Design review of the part built by this model. Coordinates are the model's own, in mm. Face numbers are marked on the shaded views. A direction names the side the tool comes from. Round coordinates to 2 decimals unless told otherwise and drop trailing zeros. Loops run counter-clockwise (first coordinate to the right, second up) from the corner with the lowest first, then second, coordinate; pieces in that order, holes last. Notation, with made-up numbers: M 27,6 L 59,6 A30 ccw 59,33 Z; hole C 84,71.5 d2. An arc over 180 degrees is marked long. Use a Markdown table: item, result.
Autodesk Inventor part; units mm, degrees
ref_plane "YZ Plane" through (0, 0, 0) normal (1, 0, 0) x (0, 1, 0)
ref_plane "XY Plane" through (0, 0, 0) normal (0, 0, 1) x (1, 0, 0)
sketch "Sketch2" plane through (0, 0, 0) normal (0, 0, 1) x (1, 0, 0)
  circle A0 centre (0, 0) radius 76.2
  dimension "d7" = 152.4
extrude "Extrusion2" add sketch "Sketch2" along normal blind 88.9
chamfer "Chamfer1" distance 19.05 angle 30 1 edges at (-76.2, 0, 88.9) measured on face at (-0.8389, -20.4706, 88.9)
chamfer "Chamfer2" distance 19.05 angle 30 1 edges at (-76.2, 0, 0) measured on face at (-0.8389, -20.4706, 0)
ref_plane "Work Plane1" through (0, -76.2, 0) normal (0, 1, 0) x (-1, 0, 0)
sketch "Sketch10" plane through (0, -76.2, 0) normal (0, 1, 0) x (-1, 0, 0)
  line L0 (88.9, 77.9015) -> (-88.9, 77.9015)
  line L1 (-88.9, 77.9015) -> (-88.9, 10.9985)
  line L2 (-88.9, 10.9985) -> (88.9, 10.9985)
  line L3 (88.9, 10.9985) -> (88.9, 77.9015)
  line L4 (-76.2, 10.9985) -> (76.2, 10.9985) construction
  line L5 (76.2, 77.9015) -> (-76.2, 77.9015) construction
  line L6 (0, -18.1203) -> (0, 108.7218) construction
  dimension "d46" = 88.9
  dimension "d47" = 88.9
extrude "Extrusion11" add sketch "Sketch10" along normal mid plane 76.2
properties part number "transmission_box_l_to_r"
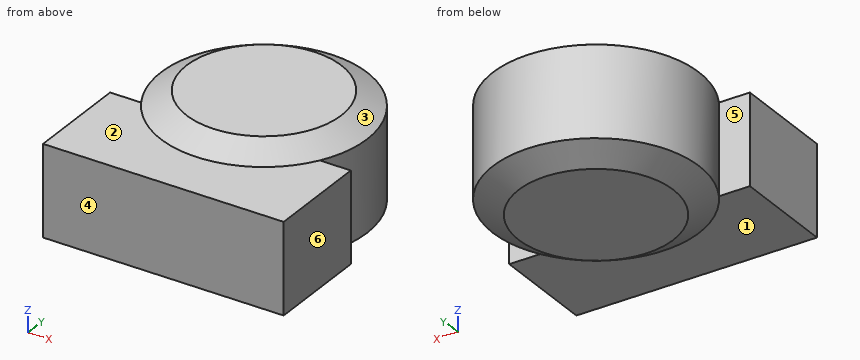
1. The part is to be moulded in two halves that separate along Y. For the marked faces 4, 5 and 6, say which applies: pulls with the +Y half, pulls with the -Y half, needs draft (parallel to the pull), parting line crosses it, or undercut.
Check values:
| item | result |
|---|---|
| face 4 | pulls with the -Y half |
| face 5 | undercut |
| face 6 | needs draft |
2. Take a section at C-C on z = 18.5. Give the boundary of the cut face in (x, y).
Check values:
| item | result |
|---|---|
| outline | M -88.9,-114.3 L 88.9,-114.3 L 88.9,-38.1 L 65.99,-38.1 A76.2 ccw long -65.99,-38.1 L -88.9,-38.1 Z |
3. Insertion check: pin 1 (5 mm diameter, centred on x = -14, z = 71.5, fed in from +Y); pin 2 (3 mm diameter, centred on y = -26, z = 24, fed in from +X); pin 3 (1.5 mm diameter, centred on x = 55, y = -71.5, fed in from -Z). Each pin has a flat end and moves straight along its axis. Give the tip position at first contact, or say it passes through.
Check values:
| item | result |
|---|---|
| pin 1 | stops at y = 75.33 |
| pin 2 | stops at x = 72.15 |
| pin 3 | stops at z = 11 |
4. Wall thickness on line 1 along Y through (x, z) = (-1.5, 24.5); line 2 along Y through (x, z) = (-80, 23); line 3 along X through (y, z) = (1.5, 22.5): over which ranges is each line inside the solid? List them lowest first. Write a range as from..to.
Check values:
| item | result |
|---|---|
| line 1 | y = -114.3..76.19 |
| line 2 | y = -114.3..-38.1 |
| line 3 | x = -76.19..76.19 |
5. Machinability: for the marked faces 1, 2 and 3, which of the approach directions +Z, -Z, +X, -X, +Y, -Y give a long, thin tool a straight path to every point of the face, cutting with its end or side? Answer none if there is none.
Check values:
| item | result |
|---|---|
| face 1 | -Z, -Y |
| face 2 | +Z, -Y |
| face 3 | +Z |
6. Take a section at A-A on y = 0. Give the boundary of the cut face in (x, z), and give its area (3 significant figures).
Check values:
| item | result |
|---|---|
| outline | M -76.2,11 L -57.15,0 L 57.15,0 L 76.2,11 L 76.2,77.9 L 57.15,88.9 L -57.15,88.9 L -76.2,77.9 Z |
| area | 13,100 mm² |
7. Take a section at B-B on x = 0. Give the boundary of the cut face in (y, z), and give its area (3 significant figures).
Check values:
| item | result |
|---|---|
| outline | M -114.3,11 L -76.2,11 L -57.15,0 L 57.15,0 L 76.2,11 L 76.2,77.9 L 57.15,88.9 L -57.15,88.9 L -76.2,77.9 L -114.3,77.9 Z |
| area | 15,700 mm² |
